Can you work these out from the model? Positions are in its coordinate system, mm. A direction names the side the tool comes from. Round coordinates to 2 decimals unless told otherwise and drop trailing zeros. Order: outer loops, then holes, each group sorted by start corner. A loop starts at its lowest first (then second) coordinate and runs counter-clockwise, first axis right, second up. Notation, with made-up numbers: (84.25, 0) -> (101.25, 0) arc R15 cw to (101.25, 24) -> close; hole circle Ø1 at (45, -3). An arc over 180 degrees is marked (long way). Use a Markdown table: item, result. Add a question column.
Q1. I need wall thicknesses on line 1 along Y through (x, z) = (-12, 13); line 2 along X through (y, z) = (8, -6.5); line 3 along Z through (x, y) = (17.5, 1). Which ranges of each line are inside material? Lowest first, please. Write a range as [from, to].
Q2. If we section it at D-D on z = -16.5: List the corners of the cut face in (x, y) for me, plus the area to 3 significant figures.
Q3. If we section it at B-B on x = 0: List the corners of the cut face in (y, z) for me.
Q4. We'd pull the mould along Z, two halves only. Please class faces 1 (the face through (-18, 2, 0)), 2 (the face through (-5, 4, 0)), 3 (the face through (0, 6.5, -9.9)): +Z half, -Z half, draft (parallel to the pull), parting line (faces both ways), or undercut.
Q5. For faces 4 (the face through (1.9, 6, 0)), 5 (the face through (0, 6.5, 9.9)), 6 (the face through (-1.9, 6, 0)), 7 (the face through (0, 2, -18)), which set-ups out of +Z, -Z, +X, -X, +Y, -Y let a thin tool reach every point of the face, with its end or its side?
Q6. If we section it at A-A on z = 0: List the corners of the cut face in (x, y) for me.
Q7. I'm going to push flat-ended pins straight in: pin 1 Ø4 at (y, z) = (4.5, -18) entering from -X; pin 2 Ø1.5 at (y, z) = (6, -3.5) entering from +X; pin 3 Ø3 at (y, z) = (5, -2.5) entering from +X; pin 4 Ø22.5 at (x, z) = (7.5, 1) entering from +Y. Where does each tip first touch, or does it pass through?
Q8. If we section it at C-C on y = 2.75: List the corners of the cut face in (x, z) for me, plus the area to 3 significant figures.
Autodesk Inventor part; units mm, degrees
ref_plane "YZ Plane" through (0, 0, 0) normal (1, 0, 0) x (0, 1, 0)
ref_plane "XZ Plane" through (0, 0, 0) normal (0, 1, 0) x (-1, 0, 0)
ref_plane "XY Plane" through (0, 0, 0) normal (0, 0, 1) x (1, 0, 0)
sketch "Sketch1" plane through (0, 0, 0) normal (0, 1, 0) x (-1, 0, 0)
  circle A0 centre (0, 0) radius 22.5
  dimension "d0" = 45
extrude "Extrusion1" add sketch "Sketch1" along normal blind 4
sketch "Sketch2" plane through (0, 4, 0) normal (0, 1, 0) x (1, 0, 0)
  line L0 (0, 0) -> (0, 8) construction
  line L1 (0, 0) -> (0, -8) construction
  circle A0 centre (0, 8) radius 1.9
  circle A1 centre (0, 0) radius 1.9
  circle A2 centre (0, -8) radius 1.9
  line L2 (1.9, 0) -> (1.9, -8)
  line L3 (1.9, 0) -> (1.9, 8)
  line L4 (-1.9, -8) -> (-1.9, 0)
  line L5 (-1.9, 0) -> (-1.9, 8)
  dimension "d3" = 8
  dimension "d4" = 8
  dimension "d5" = 3.8
  dimension "d6" = 3.8
  dimension "d7" = 3.8
extrude "Extrusion2" add sketch "Sketch2" along normal blind 5
sketch "Sketch7" plane through (0, 0, 0) normal (0, -1, 0) x (1, 0, 0)
  circle A0 centre (0, 0) radius 16.5 construction
  circle A1 centre (0, 16.5) radius 1.5
  circle A2 centre (16.5, 0) radius 1.5
  circle A3 centre (-16.5, 0) radius 1.5
  circle A4 centre (0, -16.5) radius 1.5
  dimension "d42" = 33
  dimension "d43" = 3
  dimension "d44" = 3
  dimension "d45" = 3
  dimension "d46" = 3
extrude "Extrusion6" cut sketch "Sketch7" against normal blind 5
properties part number "motormount_v3_richard"
Answer below:
| question | item | result |
|---|---|---|
| 1 | line 1 | [0, 4] |
| 1 | line 2 | [-1.9, 1.9] |
| 1 | line 3 | [-14.14, -1.12], [1.12, 14.14] |
| 2 | outline | (-15.3, 0) -> (-1.5, 0) -> (-1.5, 4) -> (-15.3, 4) -> close; (1.5, 0) -> (15.3, 0) -> (15.3, 4) -> (1.5, 4) -> close |
| 2 | area | 110 mm² |
| 3 | outline | (0, -22.5) -> (4, -22.5) -> (4, -18) -> (0, -18) -> close; (0, -15) -> (4, -15) -> (4, -9.9) -> (9, -9.9) -> (9, 9.9) -> (4, 9.9) -> (4, 15) -> (0, 15) -> close; (0, 18) -> (4, 18) -> (4, 22.5) -> (0, 22.5) -> close |
| 4 | face 1 | undercut |
| 4 | face 2 | draft |
| 4 | face 3 | -Z half |
| 5 | face 4 | +Z, -Z, +X, +Y |
| 5 | face 5 | +Z, +Y |
| 5 | face 6 | +Z, -Z, -X, +Y |
| 5 | face 7 | +Y, -Y |
| 6 | outline | (-22.5, 0) -> (-18, 0) -> (-18, 4) -> (-22.5, 4) -> close; (-15, 0) -> (15, 0) -> (15, 4) -> (1.9, 4) -> (1.9, 9) -> (-1.9, 9) -> (-1.9, 4) -> (-15, 4) -> close; (18, 0) -> (22.5, 0) -> (22.5, 4) -> (18, 4) -> close |
| 7 | pin 1 | x = -15.75 |
| 7 | pin 2 | x = 1.9 |
| 7 | pin 3 | x = 22.46 |
| 7 | pin 4 | y = 9 |
| 8 | outline | circle Ø45 at (0, 0); hole circle Ø3 at (-16.5, 0); hole circle Ø3 at (0, -16.5); hole circle Ø3 at (0, 16.5); hole circle Ø3 at (16.5, 0) |
| 8 | area | 1,560 mm² |
